Part model, mm, in its own coordinate system. Face numbers are marked on the shaded views. A direction names the side the tool comes from. Coordinates: 2 decimals unless noted, no trailing zeros. Order: outer loops, then holes, each group sorted by start corner. A loop starts at its lowest first (then second) coordinate and runs counter-clockwise, first axis right, second up. Notation, with made-up numbers: (36.25, 86.5) - (74.25, 86.5) arc R15 cw to (74.25, 99.5) - close; hole circle Ø8 at (68, -19.75). An arc over 180 degrees is marked (long way). Use a Markdown table: item, result. Add a question column.
1) Wall check: L1, parallel to Y at x = -23.94, z = 1.15; L2, parallel to Y at x = -4, z = 17; L3, parallel to Y at x = 23.5, z = 2.5. Give the ranges that are in metal, low to high. Write a range as [from, to].
2) Tool access for the marked faces 5, 6, 7 and 8: list every direction of +Z, -Z, +X, -X, +Y, -Y with a clear straight run to the whole face (end or side of a thin tool).
3) Saw through at D-D on x = 9. List the corners of the cut face in (y, z).
4) Two-plate mould, pull along Y, no slides. Class the marked faces 1, 2, 3 and 4: +Y half, -Y half, draft (parallel to the pull), parting line (faces both ways), or undercut.
5) Drop flat-ended pins along their axis: P1, Ø10, axis at x = -17.5, y = -10.5, coming from the -Z side; P2, Ø5.5, axis at y = -24, z = 10, coming from the -X side; P3, Ø8, axis at x = -18.5, z = 15.5, coming from the +Y side; P4, Ø7.5, axis at y = 24.5, z = 12, coming from the +X side. Give the stop position or say it passes through.
6) Saw through at A-A on x = 23.94. List the corners of the cut face in (y, z).
7) Saw through at B-B on z = 9.25. List the corners of the cut face in (x, y).
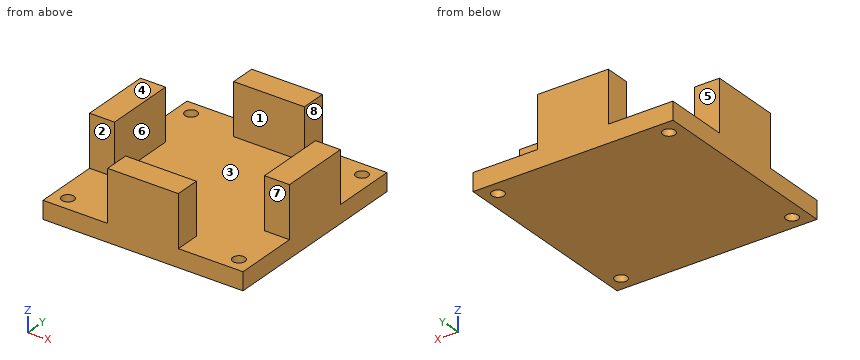
Autodesk Fusion 360 part; units mm, degrees
sketch "Sketch1" plane through (0, 0, 0) normal (0, 0, 1) x (1, 0, 0)
  line L0 (28, 28) -> (-28, 28)
  line L1 (-28, 28) -> (-28, -28)
  line L2 (-28, -28) -> (28, -28)
  line L3 (28, -28) -> (28, 28)
  line L4 (28, 28) -> (-28, -28) construction
  line L5 (-28, 28) -> (28, -28) construction
  line L6 (21, 21) -> (-21, 21)
  line L7 (-21, 21) -> (-21, -21)
  line L8 (-21, -21) -> (21, -21)
  line L9 (21, -21) -> (21, 21)
  line L10 (21, 21) -> (-21, -21) construction
  line L11 (-21, 21) -> (21, -21) construction
  line L12 (-28, 0) -> (28, 0) construction
  line L13 (0, 28) -> (0, -28) construction
  line L14 (-28, 9.9) -> (-21, 9.9)
  line L15 (-21, 9.9) -> (-21, -9.9)
  line L16 (-21, -9.9) -> (-28, -9.9)
  line L17 (-28, -9.9) -> (-28, 9.9)
  line L18 (21, -9.9) -> (28, -9.9)
  line L19 (28, 9.9) -> (21, 9.9)
  line L20 (-9.9, -28) -> (9.9, -28)
  line L21 (9.9, -28) -> (9.9, -21)
  line L22 (9.9, -21) -> (-9.9, -21)
  line L23 (-9.9, -21) -> (-9.9, -28)
  line L24 (9.9, 28) -> (9.9, 21)
  line L25 (-9.9, 21) -> (-9.9, 28)
  circle A0 centre (23.94, 23.94) radius 1.7
  circle A1 centre (-23.94, 23.94) radius 1.7
  circle A2 centre (23.94, -23.94) radius 1.7
  circle A3 centre (-23.94, -23.94) radius 1.7
  dimension "d1" = 56
  dimension "d2" = 56
  dimension "d3" = 42
  dimension "d4" = 42
  dimension "d5" = 19.8
  dimension "d6" = 19.8
  dimension "d7" = 3.4
  dimension "d8" = 4.06
  dimension "d9" = 7
sketch "Sketch2" plane through (0, 0, 0) normal (0, 1, 0) x (1, 0, 0)
  point P0 (0, -5)
  point P1 (0, -19.4)
  dimension "d10" = 5
  dimension "d11" = 14.4
extrude "Extrude1" add sketch "Sketch1" along normal up to surface (5 mm away)
extrude "Extrude2" add sketch "Sketch1" along normal up to surface (14.4 mm away) from surface at 5 contours L0 L6 L24 L25 | L3 L9 L18 L19 | L1 L7 L14 L15 L16 L17 | L2 L8 L20 L21 L22 L23
equation "d6 = d5"
equation "d8 = 0.29 * ( d1 - d3 )"
Results are:
| question | item | result |
|---|---|---|
| 1 | L1 | [-28, -25.64], [-22.24, 22.24], [25.64, 28] |
| 1 | L2 | [-28, -21], [21, 28] |
| 1 | L3 | [-28, -25.58], [-22.3, 22.3], [25.58, 28] |
| 2 | face 5 | +Z, +X, -X, +Y |
| 2 | face 6 | +Z, +Y, -Y |
| 2 | face 7 | +Z, +X, -X, -Y |
| 2 | face 8 | +Z, +X, +Y, -Y |
| 3 | outline | (-28, 0) - (28, 0) - (28, 19.4) - (21, 19.4) - (21, 5) - (-21, 5) - (-21, 19.4) - (-28, 19.4) - close |
| 4 | face 1 | undercut |
| 4 | face 2 | -Y half |
| 4 | face 3 | undercut |
| 4 | face 4 | draft |
| 5 | P1 | z = 0 |
| 5 | P2 | x = -9.9 |
| 5 | P3 | y = 9.9 |
| 5 | P4 | x = 9.9 |
| 6 | outline | (-28, 0) - (-25.64, 0) - (-25.64, 5) - (-28, 5) - close; (-22.24, 0) - (22.24, 0) - (22.24, 5) - (9.9, 5) - (9.9, 19.4) - (-9.9, 19.4) - (-9.9, 5) - (-22.24, 5) - close; (25.64, 0) - (28, 0) - (28, 5) - (25.64, 5) - close |
| 7 | outline | (-28, -9.9) - (-21, -9.9) - (-21, 9.9) - (-28, 9.9) - close; (-9.9, -28) - (9.9, -28) - (9.9, -21) - (-9.9, -21) - close; (-9.9, 21) - (9.9, 21) - (9.9, 28) - (-9.9, 28) - close; (21, -9.9) - (28, -9.9) - (28, 9.9) - (21, 9.9) - close |
